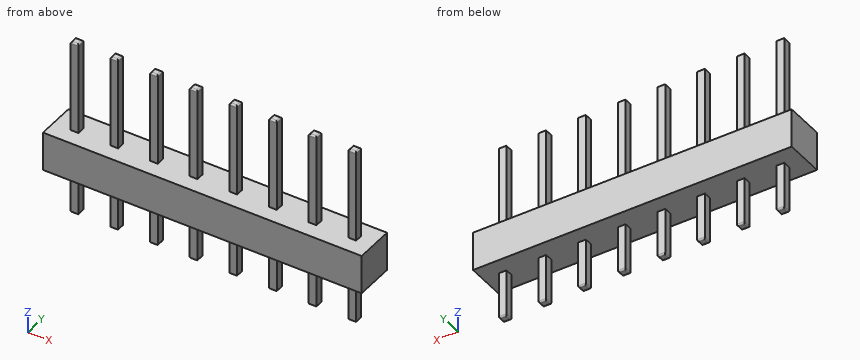
```python
from build123d import *

# Parameters (mm, degrees)
SKETCH1_W              = 20.4
SKETCH1_H              = 2.5
BOSS_EXTRUDE1_DEPTH    = 2.5
SKETCH2_W              = 0.5
SKETCH2_H              = 0.5
BOSS_EXTRUDE2_DEPTH    = 5.9
FILLET1_R              = 0.1
LPATTERN1_COUNT        = 8
LPATTERN1_PITCH        = 2.54
FILLET1_OF_LPATTERN1_R = 0.1
SKETCH4_W              = 0.5
SKETCH4_H              = 0.5
BOSS_EXTRUDE3_DEPTH    = 3
FILLET2_R              = 0.1
LPATTERN2_COUNT        = 8
LPATTERN2_PITCH        = 2.54
FILLET2_OF_LPATTERN2_R = 0.1


with BuildPart() as part:
    # Sketch1 → Boss-Extrude1 (new body)
    with BuildSketch(Plane.XY):
        Rectangle(SKETCH1_W, SKETCH1_H)
    extrude(amount=BOSS_EXTRUDE1_DEPTH)

    # Sketch2 → Boss-Extrude2 (add)
    with BuildSketch(Plane.XY.offset(2.5)):
        with Locations((8.95, 0)):
            Rectangle(SKETCH2_W, SKETCH2_H)
    boss_extrude2 = extrude(amount=BOSS_EXTRUDE2_DEPTH)

    # Fillet1
    fillet1_edges = [part.edges().sort_by_distance(p)[0] for p in [
        (9.2, 0, 8.4),
        (8.95, 0.25, 8.4),
        (8.7, 0, 8.4),
        (8.95, -0.25, 8.4),
    ]]
    fillet(fillet1_edges, radius=FILLET1_R)

    # LPattern1: Boss-Extrude2 ×8
    with Locations(*[(-i * LPATTERN1_PITCH, 0, 0) for i in range(1, LPATTERN1_COUNT)]):
        add(boss_extrude2)

    # Fillet1 of LPattern1
    fillet1_of_lpattern1_edges = [part.edges().sort_by_distance(p)[0] for p in [
        (6.66, 0, 8.4),
        (6.41, 0.25, 8.4),
        (6.16, 0, 8.4),
        (6.41, -0.25, 8.4),
        (4.12, 0, 8.4),
        (3.87, 0.25, 8.4),
        (3.62, 0, 8.4),
        (3.87, -0.25, 8.4),
        (1.58, 0, 8.4),
        (1.33, 0.25, 8.4),
        (1.08, 0, 8.4),
        (1.33, -0.25, 8.4),
        (-0.96, 0, 8.4),
        (-1.21, 0.25, 8.4),
        (-1.46, 0, 8.4),
        (-1.21, -0.25, 8.4),
        (-3.5, 0, 8.4),
        (-3.75, 0.25, 8.4),
        (-4, 0, 8.4),
        (-3.75, -0.25, 8.4),
        (-6.04, 0, 8.4),
        (-6.29, 0.25, 8.4),
        (-6.54, 0, 8.4),
        (-6.29, -0.25, 8.4),
        (-8.58, 0, 8.4),
        (-8.83, 0.25, 8.4),
        (-9.08, 0, 8.4),
        (-8.83, -0.25, 8.4),
    ]]
    fillet(fillet1_of_lpattern1_edges, radius=FILLET1_OF_LPATTERN1_R)

    # Sketch4 → Boss-Extrude3 (add)
    with BuildSketch(Plane(origin=(0, 0, 0), x_dir=(-1, 0, 0), z_dir=(0, 0, -1))):
        with Locations((-8.95, 0)):
            Rectangle(SKETCH4_W, SKETCH4_H)
    boss_extrude3 = extrude(amount=BOSS_EXTRUDE3_DEPTH)

    # Fillet2
    fillet2_edges = [part.edges().sort_by_distance(p)[0] for p in [
        (8.95, 0.25, -3),
        (9.2, 0, -3),
        (8.95, -0.25, -3),
        (8.7, 0, -3),
    ]]
    fillet(fillet2_edges, radius=FILLET2_R)

    # LPattern2: Boss-Extrude3 ×8
    with Locations(*[(-i * LPATTERN2_PITCH, 0, 0) for i in range(1, LPATTERN2_COUNT)]):
        add(boss_extrude3)

    # Fillet2 of LPattern2
    fillet2_of_lpattern2_edges = [part.edges().sort_by_distance(p)[0] for p in [
        (6.41, 0.25, -3),
        (6.66, 0, -3),
        (6.41, -0.25, -3),
        (6.16, 0, -3),
        (3.87, 0.25, -3),
        (4.12, 0, -3),
        (3.87, -0.25, -3),
        (3.62, 0, -3),
        (1.33, 0.25, -3),
        (1.58, 0, -3),
        (1.33, -0.25, -3),
        (1.08, 0, -3),
        (-1.21, 0.25, -3),
        (-0.96, 0, -3),
        (-1.21, -0.25, -3),
        (-1.46, 0, -3),
        (-3.75, 0.25, -3),
        (-3.5, 0, -3),
        (-3.75, -0.25, -3),
        (-4, 0, -3),
        (-6.29, 0.25, -3),
        (-6.04, 0, -3),
        (-6.29, -0.25, -3),
        (-6.54, 0, -3),
        (-8.83, 0.25, -3),
        (-8.58, 0, -3),
        (-8.83, -0.25, -3),
        (-9.08, 0, -3),
    ]]
    fillet(fillet2_of_lpattern2_edges, radius=FILLET2_OF_LPATTERN2_R)


solid = part.part
```
The model under review builds one solid part; all positions refer to its coordinate system, in mm. Round coordinates to 2 decimals unless told otherwise and drop trailing zeros. Order: outer loops, then holes, each group sorted by start corner. A loop starts at its lowest first (then second) coordinate and runs counter-clockwise, first axis right, second up. Notation, with made-up numbers: (77, -18) - (104, -18) arc R33 cw to (104, 20) - close; hole circle Ø4 at (2.25, -9.75). An arc over 180 degrees is marked (long way). Answer in a Markdown table with one row per item.
(1) Clearance check with flat-ended pins moving along their axes: P1, Ø0.6, axis at x = -6, z = 5, coming from the -Y side; P2, Ø0.6, axis at y = 0, z = -1, coming from the -X side; P3, Ø1.5, axis at y = -0.5, z = 5.5, coming from the +X side. State where each tip first meets the part, or that it passes through.
Result set:
| item | result |
|---|---|
| P1 | stops at y = -0.25 |
| P2 | stops at x = -9.08 |
| P3 | stops at x = 9.2 |
(2) For line 1 (Z direction, x = 7.25, y = -0.3), list the stretches that pass through material, from the lowest coordinate up. Write a range as from..to.
Result set:
| item | result |
|---|---|
| line 1 | z = 0..2.5 |
(3) Take a section at A-A on z = -1.5. Count the separate pieces of the cut face and the enclosed holes in it, plus the area to 3 significant figures.
Result set:
| item | result |
|---|---|
| separate pieces | 8 |
| enclosed holes | 0 |
| area | 2.00 mm2 |
(4) Take a section at C-C on y = 0.75. Write out the cut boundary in (x, z), plus the area to 3 significant figures.
Result set:
| item | result |
|---|---|
| outline | (-10.2, 0) - (10.2, 0) - (10.2, 2.5) - (-10.2, 2.5) - close |
| area | 51.0 mm2 |
(5) Take a section at B-B on x = -8. Write out the cut boundary in (y, z), plus the area to 3 significant figures.
Result set:
| item | result |
|---|---|
| outline | (-1.25, 0) - (1.25, 0) - (1.25, 2.5) - (-1.25, 2.5) - close |
| area | 6.25 mm2 |
